Study the drawing (mm; zero at the part's minimum x, y, z) and answer. A direction names the side the tool comes from. Coordinates: 2 decimals unless noted, no trailing zeros. Loops run counter-clockwise (first coordinate to the right, second up) from the corner with the lowest first, then second, coordinate; pieces in that order, holes last. Notation, with made-up numbers: (41.25, 13.25) -> (85.25, 13.25) arc R19 ccw to (85.25, 21.25) -> close; hole circle Ø4 at (-28, 0). An arc over 180 degrees is marked (long way). One line per question, with ' | ' between items.
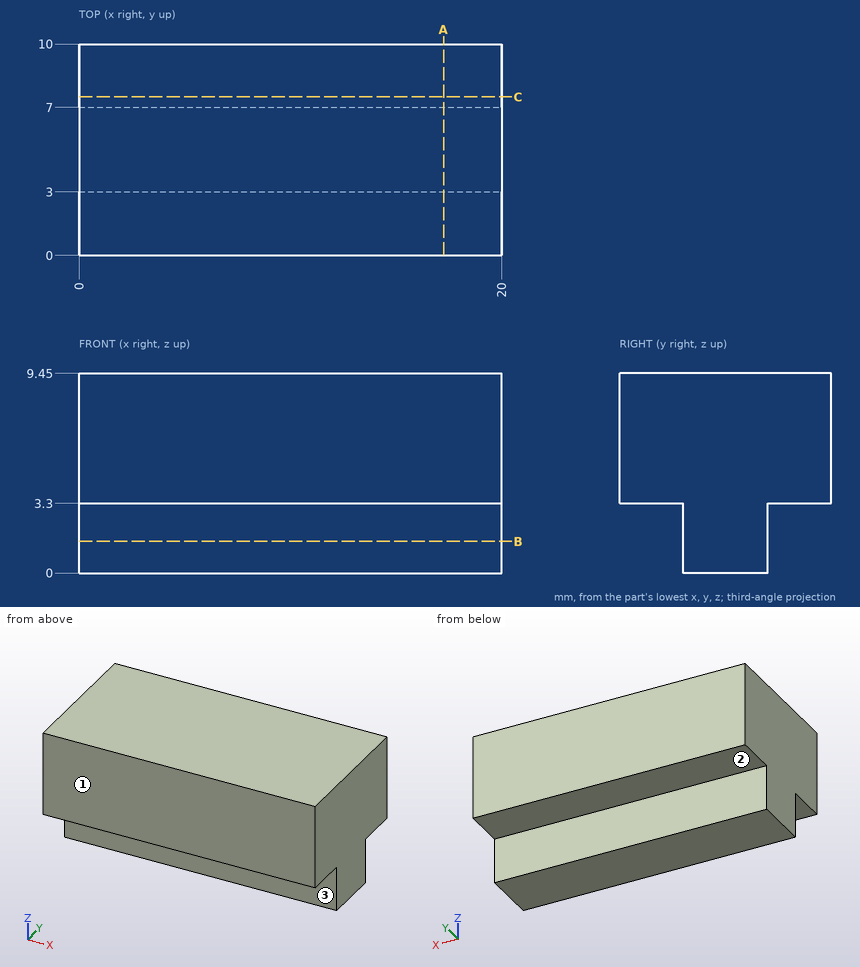
1) Find section A-A (x = 17.25). Write down the section's boundary in (y, z).
Check values:
outline: (0, 3.3) -> (3, 3.3) -> (3, 0) -> (7, 0) -> (7, 3.3) -> (10, 3.3) -> (10, 9.45) -> (0, 9.45) -> close
2) For the marked faces 1, 2 and 3, determine the directions among +Z, -Z, +X, -X, +Y, -Y from which every point of the face is accessible in a straight line to the end or side of a thin tool.
Check values:
face 1: +Z, -Z, +X, -X, -Y | face 2: -Z, +X, -X, +Y | face 3: -Z, +X, -X, -Y
3) Find the intervals of material crossed by line 1 along Z through (x, y) = (8.75, 0.75); line 2 along Y through (x, z) = (16.25, 2.25), in increasing order.
Check values:
line 1: z = 3.3 to 9.45 | line 2: y = 3 to 7
4) Find section B-B (z = 1.5). Write down the section's boundary in (x, y), plus the area to 3 significant figures.
Check values:
outline: (0, 3) -> (20, 3) -> (20, 7) -> (0, 7) -> close | area: 80.0 mm^2
5) Flat-ended cylindrical pins translate along their axes: pin 1 (2.5 mm diameter, centred on x = 12, z = 1.5, fed in from +Y); pin 2 (1 mm diameter, centred on x = 4, y = 7, fed in from -Z); pin 3 (1.6 mm diameter, centred on x = 14, z = 1.5, fed in from -Y). Find the tip coordinate at first contact, or state that the pin passes through.
Check values:
pin 1: stops at y = 7 | pin 2: stops at z = 0 | pin 3: stops at y = 3
6) Find section C-C (y = 7.5). Write down the section's boundary in (x, z).
Check values:
outline: (0, 3.3) -> (20, 3.3) -> (20, 9.45) -> (0, 9.45) -> close
